Check sheet for the modelled part. Datum: model origin and axes. Units: mm. Coordinates: 2 decimals unless noted, no trailing zeros. Loops run counter-clockwise (first coordinate to the right, second up) from the corner with the lowest first, then second, coordinate; pieces in that order, holes last.
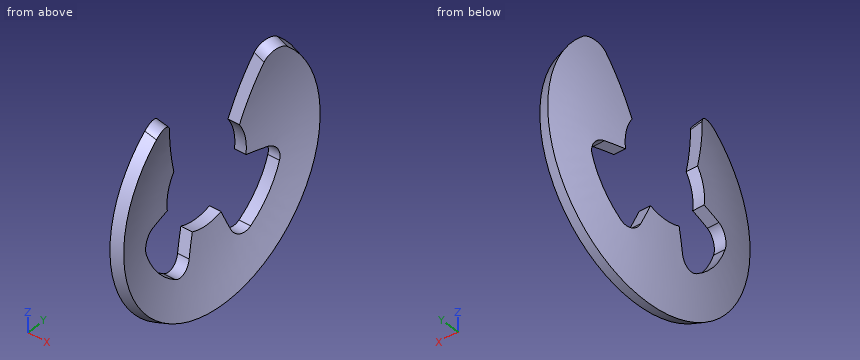
from build123d import *

# Parameters (mm, degrees)
CUT_EXTRUDE1_DEPTH = 10.608101884
FILLET1_R          = 0.762


with BuildPart() as part:
    # Sketch2 → Revolve1 (revolve)
    with BuildSketch(Plane(origin=(0, 0, 0), x_dir=(1, 0, 0), z_dir=(0, 1, 0)), mode=Mode.PRIVATE) as revolve1_sk:
        with BuildLine():
            Line((0.41129695, 6.6929), (1.016, 6.499097983))
            ThreePointArc((1.016, 6.499097983), (0.255533191, 3.289016973), (0, 0))
            Line((0, 0), (-0.635, 0))
            ThreePointArc((-0.635, 0), (-0.371846852, 3.38709491), (0.41129695, 6.6929))
        make_face()
    revolve(revolve1_sk.sketch.rotate(Axis((0, 0, 0), (1, 0, 0)), 180), axis=Axis((0, 0, 0), (1, 0, 0)))

    # Sketch1 → Cut-Extrude1 (cut, through all)
    with BuildSketch(Plane(origin=(1.016, 0, 0), x_dir=(0, 0, -1), z_dir=(1, 0, 0))):
        with BuildLine():
            Line((-5.711929949, -3.488375935), (-1.481934955, -2.171401391))
            ThreePointArc((-1.481934955, -2.171401391), (-0.600870128, -2.559310512), (0.360768614, -2.604027883))
            Line((0.360768614, -2.604027883), (0.639623582, -4.616803059))
            ThreePointArc((0.639623582, -4.616803059), (2.89470911, -3.653032709), (4.34839739, -1.677924))
            Line((4.34839739, -1.677924), (2.45263831, -0.946404))
            ThreePointArc((2.45263831, -0.946404), (2.6289, 0), (2.45263831, 0.946404))
            Line((2.45263831, 0.946404), (4.34839739, 1.677924))
            ThreePointArc((4.34839739, 1.677924), (2.89470911, 3.653032709), (0.639623582, 4.616803059))
            Line((0.639623582, 4.616803059), (0.360768614, 2.604027883))
            ThreePointArc((0.360768614, 2.604027883), (-0.600870128, 2.559310512), (-1.481934955, 2.171401391))
            Line((-1.481934955, 2.171401391), (-5.711929949, 3.488375935))
            ThreePointArc((-5.711929949, 3.488375935), (-6.6929, 0), (-5.711929949, -3.488375935))
        make_face()
    extrude(amount=-CUT_EXTRUDE1_DEPTH, mode=Mode.SUBTRACT)

    # Fillet1
    fillet1_edges = [part.edges().sort_by_distance(p)[0] for p in [
        (0.191190066, 4.616803059, -0.639623582),
        (0.191190066, 1.677924, -4.34839739),
        (0.191190066, -1.677924, -4.34839739),
        (0.191190066, -4.616803059, -0.639623582),
        (0.713662776, -3.458657833, 5.616478276),
        (0.713662776, 3.458657833, 5.616478276),
    ]]
    fillet(fillet1_edges, radius=FILLET1_R)


solid = part.part
(1) Gauge pin test, flat ends, axial feed: P1, Ø4, axis at y = 1.5, z = -2, coming from the +X side; P2, Ø4, axis at y = 0.5, z = 3, coming from the +X side; P3, Ø5, axis at y = -2.5, z = 0.5, coming from the +X side. Record the tip position at first contact, or that the pin passes through.
(2) Section check A-A, the plane z = 0. Enter the section's corners in (x, y), plus the area to 3 significant figures.
(3) Section check B-B, the plane y = 0. Enter the section's corners in (x, z).
(4) Scan lines: line 1 along X through (y, z) = (0.75, -3.75); line 2 along Y through (x, z) = (0.5, 4); line 3 along X through (y, z) = (4.75, -3.75). Record each from-to range of solid material in increasing order.
Determined:
1. P1: stops at x = 0.45
1. P2: passes through
1. P3: stops at x = 0.61
2. outline: (-0.48, -2.63) arc R21.93 ccw to (0.41, -6.69) - (1.02, -6.5) arc R21.29 cw to (0.16, -2.63) - close; (-0.48, 2.63) - (0.16, 2.63) arc R21.29 cw to (1.02, 6.5) - (0.41, 6.69) arc R21.93 ccw to start
2. area: 5.17 mm2
3. outline: (-0.48, -2.63) arc R21.93 ccw to (0.41, -6.69) - (1.02, -6.5) arc R21.29 cw to (0.16, -2.63) - close
4. line 1: x = -0.3 to 0.35
4. line 2: y = -5.33 to -2.96, 2.96 to 5.33
4. line 3: x = 0.22 to 0.88
